The model under review builds one solid part; all positions refer to its coordinate system, in mm. Face numbers are marked on the shaded views. A direction names the side the tool comes from. Give positions to 0.01 mm unless a question says otherwise; leave off trailing zeros. Write each loop counter-clockwise with the first axis right and the second up, starting at its lowest first coordinate (ties: lowest second). Pieces come first, ordered by that corner, then holes. Notation, with made-up numbers: (83, 36) - (90, 36) arc R19 cw to (90, 65) - close; hole circle Ø10 at (76, 81). An arc over 180 degrees is marked (long way). One line per question, with ' | ' between items. Start each with the question number.
```python
from build123d import *

# Parameters (mm, degrees)
SKETCH_1_W          = 7
SKETCH_1_H          = 4.5
EXTRUDE_1_DEPTH     = 1
SKETCH_1_3_W        = 7
SKETCH_1_3_H        = 5
EXTRUDE_2_DEPTH     = 4
FILLET2_R           = 2
SKETCH_2_W          = 19
SKETCH_2_H          = 5
EXTRUDE_3_DEPTH     = 2
SKETCH_2_4_W        = 19
SKETCH_2_4_H        = 5
EXTRUDE_4_DEPTH     = 2.5
SKETCH_11_W         = 1.26
SKETCH_11_H         = 5
CUT_EXTRUDE_4_DEPTH = 1.3
BOSS_EXTRUDE1_DEPTH = 6
BOSS_EXTRUDE2_DEPTH = 6
SKETCH5_R           = 0.8
CUT_EXTRUDE3_DEPTH  = 33.339752706
CUT_EXTRUDE8_DEPTH  = 27.643190595


with BuildPart() as part:
    # 草图1 → 凸台-拉伸1 (new body)
    with BuildSketch(Plane(origin=(0, 0, 0), x_dir=(1, 0, 0), z_dir=(0, 1, 0))):
        with Locations((0, 2.75)):
            Rectangle(SKETCH_1_W, SKETCH_1_H)
    extrude(amount=-EXTRUDE_1_DEPTH)

    # 草图1<3> → 凸台-拉伸2 (add)
    with BuildSketch(Plane(origin=(0, 0, 0), x_dir=(1, 0, 0), z_dir=(0, 1, 0))):
        with Locations((0, -2)):
            Rectangle(SKETCH_1_3_W, SKETCH_1_3_H)
    extrude(amount=-EXTRUDE_2_DEPTH)

    # Fillet2
    fillet2_edges = [part.edges().sort_by_distance(p)[0] for p in [
        (0, -1, -0.5),
    ]]
    fillet(fillet2_edges, radius=FILLET2_R)

    # 草图2 → 凸台-拉伸3 (add)
    with BuildSketch(Plane.XZ.offset(4)):
        with Locations((0, 2)):
            Rectangle(SKETCH_2_W, SKETCH_2_H)
    extrude(amount=EXTRUDE_3_DEPTH)

    # 草图2<4> → 凸台-拉伸4 (add)
    with BuildSketch(Plane.XZ.offset(4)):
        with Locations((0, 2)):
            Rectangle(SKETCH_2_4_W, SKETCH_2_4_H)
    extrude(amount=-EXTRUDE_4_DEPTH)

    # 草图11 → 切除-拉伸4 (cut)
    with BuildSketch(Plane(origin=(0, 0, 0), x_dir=(1, 0, 0), z_dir=(0, 1, 0))):
        with Locations((0, 2.5)):
            Rectangle(SKETCH_11_W, SKETCH_11_H)
    extrude(amount=-CUT_EXTRUDE_4_DEPTH, mode=Mode.SUBTRACT)

    # Sketch1 → Boss-Extrude1 (add)
    with BuildSketch(Plane.ZY.offset(9.5)):
        Polygon((-1.198557159, -4.790063509), (1.301442841, -0.459936491), (5.63156986, -2.959936491), (3.13156986, -7.290063509), align=None)
    extrude(amount=BOSS_EXTRUDE1_DEPTH)

    # Sketch2 → Boss-Extrude2 (add)
    with BuildSketch(Plane(origin=(9.5, 0, 0), x_dir=(0, 0, -1), z_dir=(1, 0, 0))):
        Polygon((-5.63156986, -2.959936491), (-1.301442841, -0.459936491), (1.198557159, -4.790063509), (-3.13156986, -7.290063509), align=None)
    extrude(amount=BOSS_EXTRUDE2_DEPTH)

    # Sketch5 → Cut-Extrude3 (cut, through all)
    with BuildSketch(Plane.ZY.offset(15.5)):
        with Locations((2.216506351, -3.875)):
            Circle(SKETCH5_R)
    extrude(amount=-CUT_EXTRUDE3_DEPTH, mode=Mode.SUBTRACT)

    # Sketch8 → Cut-Extrude8 (cut, through all)
    with BuildSketch(Plane.ZY.offset(9.5)):
        Polygon((-0.5, -5.193375673), (-0.5, -6), (0.897114317, -6), align=None)
        Polygon((4.5, -4.919872981), (3.876388375, -6), (4.5, -6), align=None)
    extrude(amount=-CUT_EXTRUDE8_DEPTH, mode=Mode.SUBTRACT)


solid = part.part
```
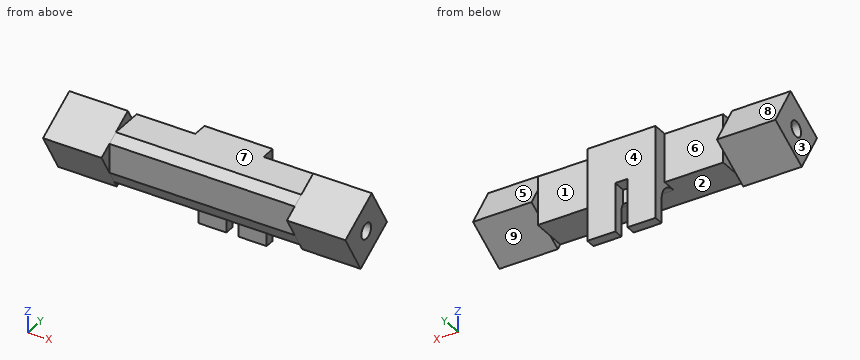
Item 1: Take a section at A-A (z = 2.25). Give the boundary of the cut face in (x, y), plus the area to 3 significant figures.
Item 2: Take a section at C-C (y = -5.5). Give the boundary of the cut face in (x, z).
Item 3: Take a section at D-D (x = 0). Give the boundary of the cut face in (y, z) (1 decimal), plus the area to 3 significant figures.
Item 4: Machinability: for the marked faces 5, 6, 7, 8 and 9, which of the approach directions +Z, -Z, +X, -X, +Y, -Y give a long, thin tool a straight path to every point of the face, cutting with its end or side? Answer none if there is none.
Item 5: Take a section at B-B (x = -8). Give the boundary of the cut face in (y, z) (1 decimal), plus the area to 3 significant figures.
Item 6: For probe 1 along Z at (x, y) = (-11, -1.5); probe 2 along Y at (x, z) = (-4.5, 2.75); probe 3 along Z at (x, y) = (-9, -3.75), list the stretches that pass through material, from the lowest coordinate up.
Item 7: The part is to be moulded in two halves that separate along X. For the marked faces 1, 2, 3 and 4, say which applies: +X half, -X half, draft (parallel to the pull), parting line (faces both ways), or undercut.
Item 8: Clearance check with flat-ended pins moving along their axes: P1, Ø3.5, axis at x = -3.5, z = 2.5, coming from the -Y side; P2, Ø1.3, axis at y = -3.88, z = 2.22, coming from the +X side; P3, Ø4, axis at x = -1, y = -3, coming from the +Z side; P4, Ø1.1, axis at x = 0, y = -3.5, coming from the -Z side. State where each tip first meets the part, or that it passes through.
Check sheet entries:
1) outline: (-15.5, -6.78) - (-9.5, -6.78) - (-9.5, -6) - (9.5, -6) - (9.5, -6.78) - (15.5, -6.78) - (15.5, -4.67) - (-15.5, -4.67) - close; (-15.5, -3.08) - (15.5, -3.08) - (15.5, -1.01) - (9.5, -1.01) - (9.5, -1.5) - (3.5, -1.5) - (3.5, 0) - (-3.5, 0) - (-3.5, -1.5) - (-9.5, -1.5) - (-9.5, -1.01) - (-15.5, -1.01) - close | area: 116 mm^2
2) outline: (-15.5, 0.03) - (15.5, 0.03) - (15.5, 4.17) - (-15.5, 4.17) - close
3) outline: (-6, 0.9) - (-5.2, -0.5) - (-3, -0.5) arc R2 cw to (-1.3, -1.4) - (-1.3, 0) - (0, 0) - (0, 4.5) - (-4.9, 4.5) - (-6, 3.9) - close; hole circle Ø1.6 at (-3.9, 2.2) | area: 26.9 mm^2
4) face 5: +Z, +X, +Y | face 6: +Z, -Z, +Y | face 7: +Z, +Y, -Y | face 8: +Z, -X, +Y | face 9: -Z, +X, +Y
5) outline: (-6, 0.9) - (-5.2, -0.5) - (-1.5, -0.5) - (-1.5, 4.5) - (-4.9, 4.5) - (-6, 3.9) - close; hole circle Ø1.6 at (-3.9, 2.2) | area: 19.6 mm^2
6) probe 1: z = 0.7 to 3.1 | probe 2: y = -6 to -4.47, -3.28 to -1.5 | probe 3: z = -0.5 to 1.43, 3.01 to 4.5
7) face 1: undercut | face 2: undercut | face 3: -X half | face 4: draft
8) P1: stops at y = -6 | P2: passes through | P3: stops at z = 4.5 | P4: stops at z = -0.5
